```python
from build123d import *

# Parameters (mm, degrees)
EXTRUDE_1_DEPTH     = 3
SKETCH_2_W          = 5
SKETCH_2_H          = 14
CUT_EXTRUDE_1_DEPTH = 10


with BuildPart() as part:
    # Эскиз1 → Бобышка-Вытянуть1 (new body)
    with BuildSketch(Plane(origin=(0, 0, 0), x_dir=(1, 0, 0), z_dir=(0, 1, 0))):
        Polygon((-12, -55), (12, -55), (12, -32), (15, -32), (15, -22), (12, -22), (12, 13), (15, 13), (15, 23), (12, 23), (12, 55), (-12, 55), (-12, 23), (-15, 23), (-15, 13), (-12, 13), (-12, -22), (-15, -22), (-15, -32), (-12, -32), align=None)
    extrude(amount=EXTRUDE_1_DEPTH)

    # Эскиз2 → Вырез-Вытянуть1 (cut)
    with BuildSketch(Plane(origin=(0, 3, 0), x_dir=(1, 0, 0), z_dir=(0, 1, 0))):
        with Locations((0, -45.4)):
            Rectangle(SKETCH_2_W, SKETCH_2_H)
    extrude(amount=-CUT_EXTRUDE_1_DEPTH, mode=Mode.SUBTRACT)


solid = part.part
```
Geometry: final body of the model. Coordinates: model frame, mm. A direction names the side the tool comes from. Round coordinates to 2 decimals unless told otherwise and drop trailing zeros. Loops run counter-clockwise (first coordinate to the right, second up) from the corner with the lowest first, then second, coordinate; pieces in that order, holes last. Notation, with made-up numbers: (34, 42.5) -> (63, 42.5) arc R27 ccw to (63, 66.5) -> close; hole circle Ø4 at (-38.75, -3.75). An arc over 180 degrees is marked (long way). Use one line per item in the form item = value. Start each with the question number.
1) Section D-D on z = 10.5. Output: boundary loops of the cut face in (x, y), then the cut area to 3 significant figures.
2) Access query for faces 5 (the flat face through (12, 1, 44)), 6 (the flat face through (-13, 1, 22)), 7 (the flat face through (14, 1, 22)), 8 (the flat face through (2.5, 2, 45)), 9 (the flat face through (-14, 1, 32)). Directions: +Z, -Z, +X, -X, +Y, -Y. A direction counts if a zero-diameter tool reaches every point of the face in a straight line with its end or side. Return the directions, or none.
3) Line query: L1, parallel to Z at x = 1.5, y = 1.85; L2, parallel to X at y = 2.15, z = 14. Output: solid intervals per line, ascending.
4) Section C-C on y = 0.8. Output: boundary loops of the cut face in (x, z), then the cut area to 3 significant figures.
5) Section B-B on z = 41. Output: boundary loops of the cut face in (x, y).
6) First-contact query: P1, Ø0.9, axis at x = -14, y = 2, coming from the +Z side; P2, Ø3, axis at x = -2, z = -21, coming from the -Y side; P3, Ø0.9, axis at y = 1, z = 43.5, coming from the -X side; P4, Ø1.5, axis at x = 13.5, y = 2, coming from the -Z side. Flat tips, straight axial feed; report the tip coordinate or a pass-through.
7) Section A-A on x = 0.5. Output: boundary loops of the cut face in (y, z).
8) Draft query along Z for faces 1 (the flat face through (14, 1, -23)), 2 (the flat face through (0, 0, -1)), 3 (the flat face through (13, 1, 32)), 4 (the flat face through (0, 2, 38.4)). Return one class per face: released by +Z, released by -Z, zero draft, split by the parting line, or undercut.
Response:
q1.outline = (-12, 0) -> (12, 0) -> (12, 3) -> (-12, 3) -> close
q1.area = 72.0 mm^2
q2.face_5 = +Z, +X, +Y, -Y
q2.face_6 = -X, +Y, -Y
q2.face_7 = +X, +Y, -Y
q2.face_8 = +Y, -Y
q2.face_9 = +Z, -X, +Y, -Y
q3.L1 = -55 to 38.4, 52.4 to 55
q3.L2 = -12 to 12
q4.outline = (-15, -23) -> (-12, -23) -> (-12, -55) -> (12, -55) -> (12, -23) -> (15, -23) -> (15, -13) -> (12, -13) -> (12, 22) -> (15, 22) -> (15, 32) -> (12, 32) -> (12, 55) -> (-12, 55) -> (-12, 32) -> (-15, 32) -> (-15, 22) -> (-12, 22) -> (-12, -13) -> (-15, -13) -> close; hole (-2.5, 38.4) -> (2.5, 38.4) -> (2.5, 52.4) -> (-2.5, 52.4) -> close
q4.area = 2,690 mm^2
q5.outline = (-12, 0) -> (-2.5, 0) -> (-2.5, 3) -> (-12, 3) -> close; (2.5, 0) -> (12, 0) -> (12, 3) -> (2.5, 3) -> close
q6.P1 = 32
q6.P2 = 0
q6.P3 = -12
q6.P4 = -23
q7.outline = (0, -55) -> (3, -55) -> (3, 38.4) -> (0, 38.4) -> close; (0, 52.4) -> (3, 52.4) -> (3, 55) -> (0, 55) -> close
q8.face_1 = released by -Z
q8.face_2 = zero draft
q8.face_3 = released by +Z
q8.face_4 = undercut
